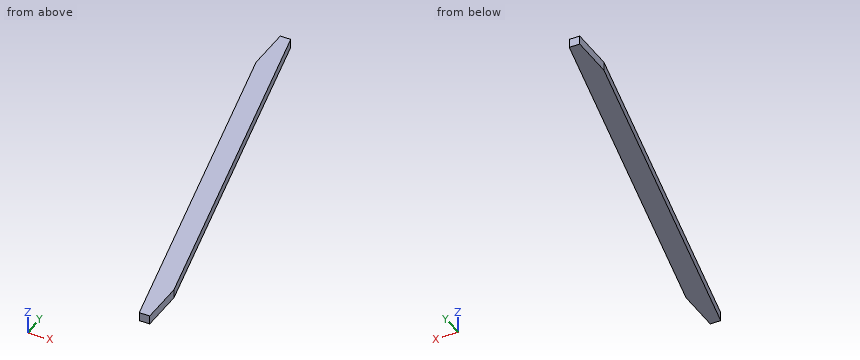
Autodesk Inventor part; units mm, degrees
ref_plane "YZ Plane" through (0, 0, 0) normal (1, 0, 0) x (0, 1, 0)
ref_plane "XZ Plane" through (0, 0, 0) normal (0, 1, 0) x (-1, 0, 0)
ref_plane "XY Plane" through (0, 0, 0) normal (0, 0, 1) x (1, 0, 0)
sketch "Sketch1" plane through (0, 0, 0) normal (0, 0, 1) x (1, 0, 0)
  line L0 (88.9, 914.4) -> (2349.5, 914.4)
  line L1 (88.9, -914.4) -> (88.9, 914.4)
  line L2 (88.9, -914.4) -> (2349.5, -914.4)
  line L3 (520.7, -914.4) -> (520.7, 914.4)
  line L4 (2349.5, -914.4) -> (2349.5, 914.4)
  line L5 (1917.7, 914.4) -> (1917.7, -914.4)
  line L6 (520.7, 743.6248) -> (520.7, -914.4)
  line L7 (88.9, -720.9648) -> (88.9, 914.4)
  line L8 (1917.7, 720.9648) -> (2303.8278, -914.4)
  line L9 (2349.5, -720.9648) -> (1963.3722, 914.4)
  line L10 (88.9, 914.4) -> (520.7, 914.4)
  line L11 (88.9, 914.4) -> (520.7, 914.4)
  line L12 (2303.8278, -914.4) -> (2349.5, -914.4)
  line L13 (2349.5, -720.9648) -> (2349.5, -914.4)
  line L14 (1917.7, 720.9648) -> (1917.7, 914.4)
  line L15 (1917.7, 914.4) -> (1963.3722, 914.4)
  line L16 (520.7, -914.4) -> (88.9, -914.4)
  line L17 (88.9, -914.4) -> (88.9, -720.9648)
  line L18 (88.9, 914.4) -> (520.7, 914.4)
  line L19 (520.7, 738.408) -> (520.7, 914.4)
  point P0 (0, 0)
extrude "Extrusion1" add sketch "Sketch1" against normal blind 38.1 contours L0 L9 L4 L2 L8 L5
properties part number "fside1"
Verification items for the finished model (mm, model axes). Coordinates: 2 decimals unless noted, no trailing zeros. Loops run counter-clockwise (first coordinate to the right, second up) from the corner with the lowest first, then second, coordinate; pieces in that order, holes last. Notation, with made-up numbers: (-16, 18.5) - (-10, 18.5) arc R18 ccw to (-10, 41.5) - close; hole circle Ø1 at (19.5, 85). An arc over 180 degrees is marked (long way). Put each result on its own line as item: value.
Item 1: Section check A-A (z = -7). Enter the section's corners in (x, y), then the cut area to 3 significant figures.
Conclusion:
outline: (1917.7, 720.96) - (2303.83, -914.4) - (2349.5, -914.4) - (2349.5, -720.96) - (1963.37, 914.4) - (1917.7, 914.4) - close
area: 158,000 mm2
Item 2: Section check B-B (x = 2028.5). Enter the section's corners in (y, z).
Conclusion:
outline: (251.69, -38.1) - (638.56, -38.1) - (638.56, 0) - (251.69, 0) - close
Item 3: Section check C-C (y = -414). Enter the section's corners in (x, z), then the cut area to 3 significant figures.
Conclusion:
outline: (2185.68, -38.1) - (2277.02, -38.1) - (2277.02, 0) - (2185.68, 0) - close
area: 3,480 mm2
Item 4: Scan lines: line 1 along X through (y, z) = (-176.5, -20); line 2 along X through (y, z) = (-678.5, -25.5). Record each from-to range of solid material in increasing order.
Conclusion:
line 1: x = 2129.6 to 2220.95
line 2: x = 2248.13 to 2339.47
Item 5: Gauge pin test, flat ends, axial feed: pin 1 Ø1.5 at (x, y) = (2006.5, 494) entering from +Z; pin 2 Ø10 at (y, z) = (561.5, -6) entering from +X. Record the tip position at first contact, or that the pin passes through.
Conclusion:
pin 1: stops at z = 0
pin 2: stops at x = 2047.88
